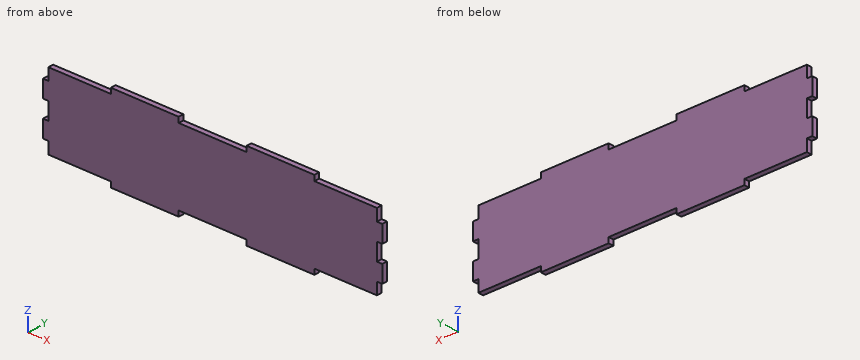
from build123d import *

# Parameters (mm, degrees)
SKETCH1_W           = 203.2
SKETCH1_H           = 50.8
BOSS_EXTRUDE1_DEPTH = 3.175
SKETCH2_W           = 40.64
SKETCH2_H           = 3.175
CUT_EXTRUDE2_DEPTH  = 3.175
LPATTERN1_COUNT     = 3
LPATTERN1_PITCH     = 81.28
SKETCH3_W           = 3.175
SKETCH3_H           = 10.16
CUT_EXTRUDE3_DEPTH  = 3.175
LPATTERN2_COUNT     = 2
LPATTERN2_PITCH     = 20.32
LPATTERN3_COUNT     = 2
LPATTERN3_PITCH     = 20.32


with BuildPart() as part:
    # Sketch1 → Boss-Extrude1 (new body)
    with BuildSketch(Plane(origin=(0, 0, 0), x_dir=(1, 0, 0), z_dir=(0, 1, 0))):
        Rectangle(SKETCH1_W, SKETCH1_H)
    extrude(amount=BOSS_EXTRUDE1_DEPTH)

    # Sketch2 → Cut-Extrude2 (cut)
    with BuildSketch(Plane(origin=(0, 3.175, 0), x_dir=(1, 0, 0), z_dir=(0, 1, 0))):
        with Locations((-81.28, 23.8125)):
            Rectangle(SKETCH2_W, SKETCH2_H)
        with Locations((-81.28, -23.8125)):
            Rectangle(SKETCH2_W, SKETCH2_H)
    cut_extrude2 = extrude(amount=-CUT_EXTRUDE2_DEPTH, mode=Mode.SUBTRACT)

    # LPattern1: Cut-Extrude2 ×3
    with Locations(*[(i * LPATTERN1_PITCH, 0, 0) for i in range(1, LPATTERN1_COUNT)]):
        add(cut_extrude2, mode=Mode.SUBTRACT)

    # Sketch3 → Cut-Extrude3 (cut)
    with BuildSketch(Plane(origin=(0, 3.175, 0), x_dir=(1, 0, 0), z_dir=(0, 1, 0))):
        with Locations((-100.0125, 0)):
            Rectangle(SKETCH3_W, SKETCH3_H)
        with Locations((100.0125, 0)):
            Rectangle(SKETCH3_W, SKETCH3_H)
    cut_extrude3 = extrude(amount=-CUT_EXTRUDE3_DEPTH, mode=Mode.SUBTRACT)

    # LPattern2: Cut-Extrude3 ×2
    with Locations(*[(0, 0, i * LPATTERN2_PITCH) for i in range(1, LPATTERN2_COUNT)]):
        add(cut_extrude3, mode=Mode.SUBTRACT)

    # LPattern3: Cut-Extrude3 ×2
    with Locations(*[(0, 0, -i * LPATTERN3_PITCH) for i in range(1, LPATTERN3_COUNT)]):
        add(cut_extrude3, mode=Mode.SUBTRACT)


solid = part.part
Read the model definition and answer for the solid it produces. Units are mm, in the model's axes. Coordinates: 2 decimals unless noted, no trailing zeros. Write each loop counter-clockwise with the first axis right and the second up, starting at its lowest first coordinate (ties: lowest second). Pieces come first, ordered by that corner, then holes. Notation, with made-up numbers: M -7,85.25 L 17,85.25 A25 cw 17,113.25 Z; hole C 87.25,-34 d9. An arc over 180 degrees is marked long. Use a Markdown table: item, result.
Q1. The part is cut by section B-B, the plane z = -3. Write down the section's boundary in (x, y) (3 decimals), then the cut area to 3 significant figures.
Answer block:
| item | result |
|---|---|
| outline | M -98.425,0 L 98.425,0 L 98.425,3.175 L -98.425,3.175 Z |
| area | 625 mm2 |
Q2. Straight lines are drawn through the part: L1, parallel to Z at x = 71.5, y = 2.8 (3 decimals); L2, parallel to X at y = 0.15, z = -23; L3, parallel to X at y = 0.5, z = -21 (3 decimals). For each, find the intervals that lie inside material, in ascending order. Write a range as [from, to].
Answer block:
| item | result |
|---|---|
| L1 | z = [-22.225, 22.225] |
| L2 | x = [-60.96, -20.32], [20.32, 60.96] |
| L3 | x = [-98.425, 98.425] |
Q3. Each of these flat-tipped pins is pushed along its axis until it touches: pin 1 Ø1 at (x, y) = (4, 1) entering from +Z (3 decimals); pin 2 Ø1 at (x, y) = (100, 2) entering from +Z; pin 3 Ø1.6 at (y, z) = (2, 24.5) entering from +X. Where does it stop, or does it pass through?
Answer block:
| item | result |
|---|---|
| pin 1 | stops at z = 22.225 |
| pin 2 | stops at z = 15.24 |
| pin 3 | stops at x = 60.96 |
Q4. The part is cut by section A-A, the plane x = 89.5. Write down the section's boundary in (y, z) (3 decimals).
Answer block:
| item | result |
|---|---|
| outline | M 0,-22.225 L 3.175,-22.225 L 3.175,22.225 L 0,22.225 Z |
